The listing builds one solid part. Answer for the finished solid, in the listing's coordinates (mm). Face numbers are marked on the shaded views. A direction names the side the tool comes from. Give positions to 0.01 mm unless a question says otherwise; leave off trailing zeros. Loops run counter-clockwise (first coordinate to the right, second up) from the corner with the lowest first, then second, coordinate; pieces in that order, holes last.
Item 1: Section D-D, the plane x = 28 is taken. Give the vertices of the cut face in (y, z), and give its area (3 significant figures).
Item 2: Section C-C, the plane z = 104 is taken. Give the number of separate pieces and of enclosed holes in the cut face, and give its area (3 significant figures).
Item 3: Section B-B, the plane y = -49.5 is taken. Give the vertices of the cut face in (x, z).
Item 4: Each of these flat-tipped pins is pushed along its axis until it touches: pin 1 Ø9.5 at (x, y) = (-57.5, 0) entering from -Z; pin 2 Ø3 at (x, z) = (-24, 59.5) entering from -Y; pin 3 Ø1 at (x, z) = (26.5, 104) entering from +Y; pin 4 Ø8 at (y, z) = (-3, 42) entering from -X. Where does it stop, or does it pass through?
Item 5: Section A-A, the plane x = -57.5 is taken. Give the vertices of the cut face in (y, z), and give its area (3 significant figures).
Item 6: The mould has two halves that part along Y. Classify the marked faces 3, 4 and 5: pulls with the +Y half, pulls with the -Y half, needs draft (parallel to the pull), parting line crosses it, or undercut.
Item 7: Consider line 1 along Z through (x, y) = (-19.5, 37); line 2 along Y through (x, z) = (-23, 105); line 3 along Y through (x, z) = (8, 16). Determine where each line is inside the solid, lowest interval first.
Item 8: A tool of negligible diameter and unlimited length cuts with its end or side. For the marked faces 1 and 2, from which of +Z, -Z, +X, -X, +Y, -Y can it reach the whole face along a straight path? Write none if from no direction.
Autodesk Fusion 360 part; units mm, degrees
sketch "Sketch1" plane through (0, 0, 0) normal (0, 0, 1) x (1, 0, 0)
  circle A0 centre (0, 0) radius 57.5
  circle A1 centre (0, 0) radius 65
  dimension "d1" = 115
  dimension "d2" = 130
extrude "Extrude1" add sketch "Sketch1" along normal blind 20 contours A0 | A1
sketch "Sketch2" plane through (0, 0, 0) normal (0, 0, -1) x (-1, 0, 0)
  circle A0 centre (0, 0) radius 65
  circle A1 centre (0, 0) radius 57.5
  circle A2 centre (0, 0) radius 47.5
  dimension "d5" = 115
  dimension "d6" = 95
extrude "Extrude2" cut sketch "Sketch2" against normal blind 3.2 contours A2
sketch "Sketch3" plane through (0, 0, 20) normal (0, 0, 1) x (1, 0, 0)
  circle A0 centre (0, 0) radius 65
  circle A1 centre (0, 0) radius 57.5
  line L0 (0, 0) -> (0, 57.5)
  dimension "d9" = 115
hole "Hole1" at (0, 57.5, 20) direction (0, 0, -1) diameter 8 end through all counterbore diameter 12 counterbore depth 9
pattern_circular "C-Pattern1" count 8 over 360 about axis through (0, 0, 1.75) along (0, 0, 1) of "Hole1"
sketch "Sketch4" plane through (0, 0, 20) normal (0, 0, 1) x (1, 0, 0)
  circle A0 centre (40.6586, 40.6586) radius 6
  circle A1 centre (57.5, 0) radius 6
  circle A2 centre (40.6586, -40.6586) radius 6
  circle A3 centre (0, -57.5) radius 6
  circle A4 centre (-40.6586, -40.6586) radius 6
  circle A5 centre (-57.5, 0) radius 6
  circle A6 centre (-40.6586, 40.6586) radius 6
  circle A7 centre (0, 57.5) radius 6
  circle A8 centre (0, 0) radius 65
  circle A9 centre (0, 0) radius 40
  dimension "d17" = 80
extrude "Extrude3" cut sketch "Sketch4" against normal blind 17 contours A9
sketch "Sketch5" plane through (0, 0, 20) normal (0, 0, 1) x (1, 0, 0)
  circle A0 centre (0, 0) radius 40
  circle A1 centre (40.6586, 40.6586) radius 6
  circle A2 centre (57.5, 0) radius 6
  circle A3 centre (40.6586, -40.6586) radius 6
  circle A4 centre (0, -57.5) radius 6
  circle A5 centre (-40.6586, -40.6586) radius 6
  circle A6 centre (-57.5, 0) radius 6
  circle A7 centre (-40.6586, 40.6586) radius 6
  circle A8 centre (0, 57.5) radius 6
  circle A9 centre (0, 0) radius 65
  circle A10 centre (0, 0) radius 47.5
  dimension "d20" = 95
extrude "Extrude4" add sketch "Sketch5" along normal blind 80 contours A10
sketch "Sketch6" plane through (0, 0, 100) normal (0, 0, 1) x (1, 0, 0)
  circle A0 centre (0, 0) radius 40
  circle A1 centre (0, 0) radius 47.5
  circle A2 centre (0, 0) radius 65
extrude "Extrude5" add sketch "Sketch6" along normal blind 20 contours A1 | A2
sketch "Sketch7" plane through (0, 0, 100) normal (0, 0, -1) x (-1, 0, 0)
  circle A0 centre (0, 0) radius 65
  circle A1 centre (0, 0) radius 47.5
  line L0 (0, 0) -> (0, 57.5)
  dimension "d25" = 57.5
hole "Hole2" at (0, 57.5, 100) direction (0, 0, 1) diameter 8 end through all counterbore diameter 12 counterbore depth 10
pattern_circular "C-Pattern2" count 8 over 360 about axis through (0, 0, 1.75) along (0, 0, 1) of "Hole2"
equation "d2 = 115 mm + 15 mm"
equation "d25 = ( 115 / 2 ) * 1 mm"
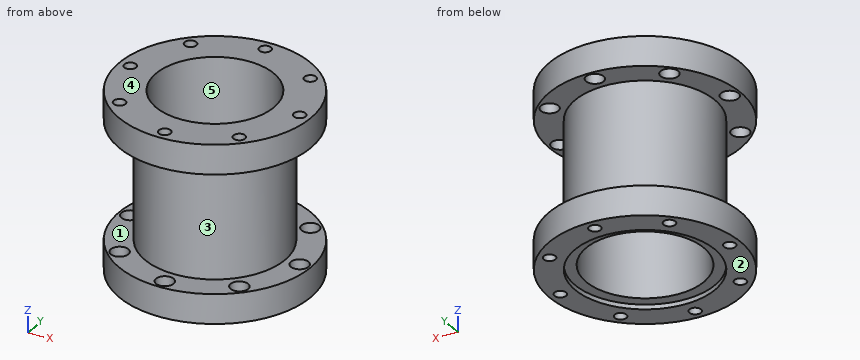
Worked answers:
1. outline: (-58.66, 0) - (-38.37, 0) - (-38.37, 3.2) - (-28.57, 3.2) - (-28.57, 120) - (-58.66, 120) - (-58.66, 100) - (-38.37, 100) - (-38.37, 20) - (-58.66, 20) - close; (28.57, 3.2) - (38.37, 3.2) - (38.37, 0) - (58.66, 0) - (58.66, 20) - (38.37, 20) - (38.37, 100) - (58.66, 100) - (58.66, 120) - (28.57, 120) - close
1. area: 3,910 mm2
2. separate pieces: 1
2. enclosed holes: 9
2. area: 7,340 mm2
3. outline: (-42.13, 0) - (42.13, 0) - (42.13, 20) - (-42.13, 20) - close; (-42.13, 100) - (42.13, 100) - (42.13, 120) - (-42.13, 120) - close
4. pin 1: stops at z = 0
4. pin 2: stops at y = -41.83
4. pin 3: stops at y = 59.57
4. pin 4: stops at x = -47.5
5. outline: (-30.31, 0) - (-4, 0) - (-4, 11) - (-6, 11) - (-6, 20) - (-30.31, 20) - close; (-30.31, 100) - (-6, 100) - (-6, 110) - (-4, 110) - (-4, 120) - (-30.31, 120) - close; (4, 0) - (30.31, 0) - (30.31, 20) - (6, 20) - (6, 11) - (4, 11) - close; (4, 110) - (6, 110) - (6, 100) - (30.31, 100) - (30.31, 120) - (4, 120) - close
5. area: 2,030 mm2
6. face 3: parting line crosses it
6. face 4: needs draft
6. face 5: undercut
7. line 1: z = 3.2 to 120
7. line 2: y = -60.79 to -32.73, 32.73 to 60.79
7. line 3: y = -64.51 to -39.19, 39.19 to 64.51
8. face 1: none
8. face 2: -Z, +X, -X, +Y, -Y
